```python
from build123d import *

# Parameters (mm, degrees)
F1_DEPTH       = 4
F3_D           = 3.3
F3_CSINK_D     = 8.96
F3_CSINK_ANGLE = 90
F4_SIZE        = 2
F5_R           = 2
F6_SIZE        = 2


with BuildPart() as f1:
    # F0 (on Top) → F1 (new body, symmetric)
    with BuildSketch(Plane.XY):
        with BuildLine():
            ThreePointArc((-4, 0), (0, 4), (4, 0))
            Line((4, 0), (4, -4))
            Line((4, -4), (15, -4))
            Line((15, -4), (15, 6))
            Line((15, 6), (0, 6))
            ThreePointArc((0, 6), (-4.2426406871, 4.2426406871), (-6, 0))
            Line((-6, 0), (-4, 0))
        make_face()
    extrude(amount=F1_DEPTH, both=True)

    # F3 (through all)
    with Locations(Plane(origin=(0, 6, 0), x_dir=(-1, 0, 0), z_dir=(0, 1, 0))):
        with Locations((-9.5, 0)):
            CounterSinkHole(F3_D / 2, F3_CSINK_D / 2, counter_sink_angle=F3_CSINK_ANGLE)

    # F4
    f4_edges = [f1.edges().sort_by_distance(p)[0] for p in [
        (15, 1, -4),
        (15, 1, 4),
    ]]
    chamfer(f4_edges, length=F4_SIZE)

    # F5
    f5_edges = [f1.edges().sort_by_distance(p)[0] for p in [
        (15, 1, 2),
        (15, 1, -2),
    ]]
    fillet(f5_edges, radius=F5_R)

    # F6
    f6_edges = [f1.edges().sort_by_distance(p)[0] for p in [
        (8.5, -4, 4),
    ]]
    chamfer(f6_edges, length=F6_SIZE)


solid = f1.part
```
Part model, mm, in its own coordinate system. A direction names the side the tool comes from. Coordinates: 2 decimals unless noted, no trailing zeros. Loops run counter-clockwise (first coordinate to the right, second up) from the corner with the lowest first, then second, coordinate; pieces in that order, holes last. Notation, with made-up numbers: (21, -37) - (60, -37) arc R23 cw to (60, -19) - close; hole circle Ø4 at (8, 12). An arc over 180 degrees is marked (long way). Write item = value, one per line. Start each with the question number.
Item 1: Wall check: L1, parallel to X at y = -2, z = 0; L2, parallel to Z at x = 9.5, y = -1.75; L3, parallel to X at y = 3, z = -0.25. Give the ranges that are in metal, low to high. Write a range as from..to.
Item 2: Cut at A-A, the plane z = 0. Give the cut face in (x, y), and give its area (3 significant figures).
Item 3: 3-axis set-ups, long thin cutter, end or side, ignore diameter. For faces 4 (the flat face through (4, -2, 0)), 5 (the cylindrical face through (0, 4, 0)): which of +Z, -Z, +X, -X, +Y, -Y reach the whole face in a straight line?
Item 4: Cut at C-C, the plane x = 9.5. Give the cut face in (y, z).
Item 5: Flat gauge pins, fed straight in: pin 1 Ø3 at (x, z) = (7.5, 2) entering from +Y; pin 2 Ø2 at (x, z) = (-4.5, 1) entering from -Y; pin 3 Ø3 at (x, z) = (11, -2.5) entering from +Y. Where does each tip first touch, or does it go through?
Item 6: Mould opens along Z. For faces 1 (the flat face through (9, -3, 3)), 2 (the flat face through (-5, 0, 0)), 3 (the conical face through (11.151, 3.307, -0.685)) say: released by +Z, released by -Z, zero draft, split by the parting line, or undercut.
Item 7: Cut at B-B, the plane y = 1.5. Give the cut face in (x, z), and give its area (3 significant figures).
Item 8: Cut at D-D, the plane y = 0.5. Give the cut face in (x, z), and give its area (3 significant figures).
The answers:
q1.L1 = 4..7.85, 11.15..15
q1.L2 = -4..-1.65, 1.65..4
q1.L3 = -5.2..-2.65, 2.65..7.87, 11.13..15
q2.outline = (-6, 0) - (-4, 0) arc R4 cw to (4, 0) - (4, -4) - (7.85, -4) - (7.85, 3.17) - (5.02, 6) - (0, 6) arc R6 ccw to start; (11.15, -4) - (15, -4) - (15, 6) - (13.98, 6) - (11.15, 3.17) - close
q2.area = 96.1 mm2
q3.face_4 = +Z, -Z, -X, -Y
q3.face_5 = +Z, -Z, -Y
q4.outline = (-4, -4) - (5.52, -4) - (3.17, -1.65) - (-4, -1.65) - close; (-4, 1.65) - (3.17, 1.65) - (5.52, 4) - (-2, 4) - (-4, 2) - close
q5.pin_1 = 5.85
q5.pin_2 = 0
q5.pin_3 = 5.94
q6.face_1 = released by +Z
q6.face_2 = zero draft
q6.face_3 = undercut
q7.outline = (-5.81, -4) - (-3.71, -4) - (-3.71, 4) - (-5.81, 4) - close; (3.71, -4) - (13, -4) - (14.41, -2.59) arc R2 ccw to (15, -1.17) - (15, 1.17) arc R2 ccw to (14.41, 2.59) - (13, 4) - (3.71, 4) - close; hole circle Ø3.3 at (9.5, 0)
q7.area = 94.4 mm2
q8.outline = (-5.98, -4) - (-3.97, -4) - (-3.97, 4) - (-5.98, 4) - close; (3.97, -4) - (13, -4) - (14.41, -2.59) arc R2 ccw to (15, -1.17) - (15, 1.17) arc R2 ccw to (14.41, 2.59) - (13, 4) - (3.97, 4) - close; hole circle Ø3.3 at (9.5, 0)
q8.area = 91.6 mm2
